Print and shaded views of the part. All mm, measured from the part's lowest x, y and z. A direction names the side the tool comes from. Give positions to 0.01 mm unless a question says otherwise; leave off trailing zeros. Loops run counter-clockwise (first coordinate to the right, second up) from the corner with the lowest first, then second, coordinate; pieces in that order, holes last. Notation, with made-up numbers: (23.25, 59) - (70.25, 59) arc R13 ccw to (70.25, 64) - close; hole circle Ø1 at (-10.75, 44). An arc over 180 degrees is marked (long way). Return JSON: item names as keys, results as strings.
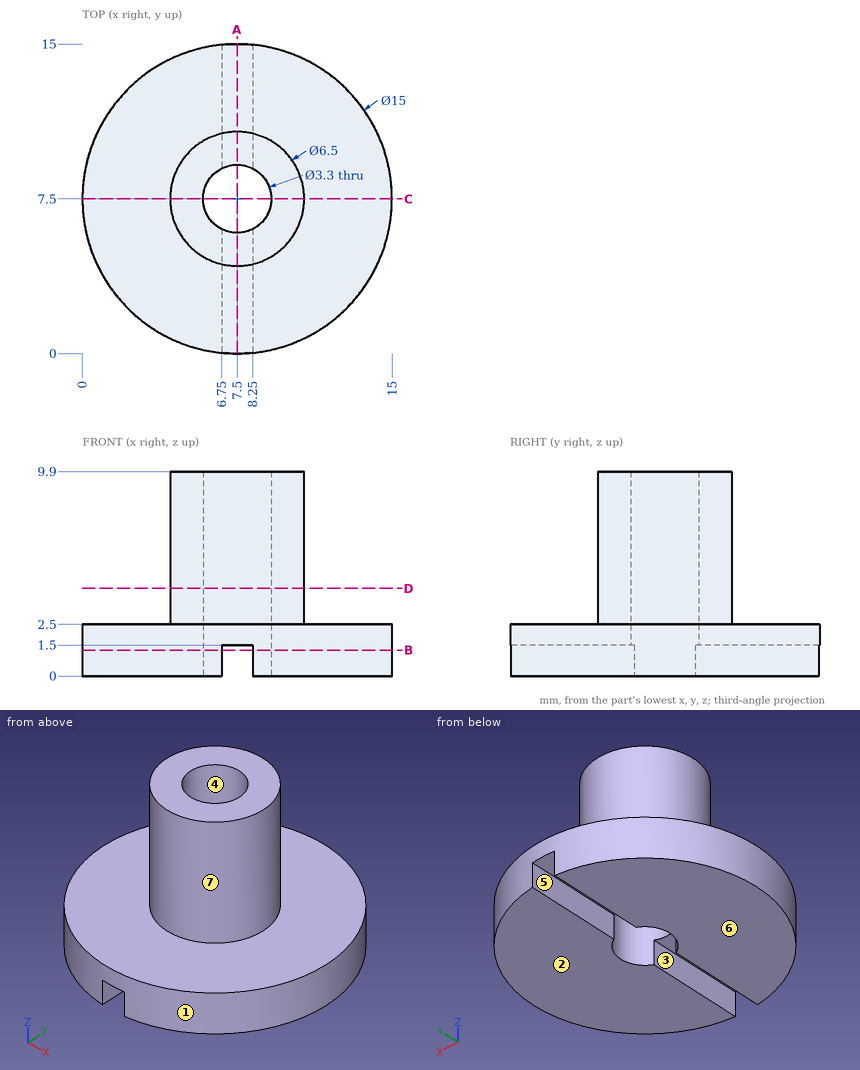
1. Which spindle directions (+Z, -Z, +X, -X, +Y, -Y) get a long thin tool onto all of the face, cutting with end or side? Do the marked faces 5, 6 and 7. Say none if no direction does.
Values follow:
{"face 5": "-Z, +Y, -Y", "face 6": "-Z, +X, -X, +Y, -Y", "face 7": "+Z"}
2. Cut at C-C, the plane y = 7.5. Write the cut outline in (x, z).
Values follow:
{"outline": "(0, 0) - (5.85, 0) - (5.85, 9.9) - (4.25, 9.9) - (4.25, 2.5) - (0, 2.5) - close; (9.15, 0) - (15, 0) - (15, 2.5) - (10.75, 2.5) - (10.75, 9.9) - (9.15, 9.9) - close"}
3. Cut at A-A, the plane x = 7.5. Write the cut outline in (y, z).
Values follow:
{"outline": "(0, 1.5) - (5.85, 1.5) - (5.85, 9.9) - (4.25, 9.9) - (4.25, 2.5) - (0, 2.5) - close; (9.15, 1.5) - (15, 1.5) - (15, 2.5) - (10.75, 2.5) - (10.75, 9.9) - (9.15, 9.9) - close"}
4. Drop flat-ended pins along their axis: P1, Ø0.8, axis at y = 11.5, z = 1, coming from the +X side; P2, Ø0.8, axis at y = 11.5, z = 0.5, coming from the -X side; P3, Ø2, axis at y = 9, z = 6.5, coming from the +X side. Give the stop position or say it passes through.
Values follow:
{"P1": "stops at x = 14.08", "P2": "stops at x = 0.92", "P3": "stops at x = 10.71"}
5. Pull direction X, two halves, no side cores. Call the marked faces 1, 2, 3 and 4: +X half, -X half, draft (parallel to the pull), parting line (faces both ways), or undercut.
Values follow:
{"face 1": "parting line", "face 2": "draft", "face 3": "undercut", "face 4": "undercut"}
6. Cut at D-D, the plane z = 4.25. Write the cut outline in (x, y), plus the area to 3 significant figures.
Values follow:
{"outline": "circle Ø6.5 at (7.5, 7.5); hole circle Ø3.3 at (7.5, 7.5)", "area": "24.6 mm²"}
7. Drill centre lines: probe 1 along Y at (x, z) = (7.5, 5.5); probe 2 along Z at (x, y) = (6.25, 1); probe 3 along Z at (x, y) = (8, 4.5). Where is each one in solid material? Low to high.
Values follow:
{"probe 1": "y = 4.25 to 5.85, 9.15 to 10.75", "probe 2": "z = 0 to 2.5", "probe 3": "z = 1.5 to 9.9"}
8. Cut at B-B, the plane z = 1.25. Write the cut outline in (x, y).
Values follow:
{"outline": "(6.75, 0.04) - (6.75, 6.03) arc R1.65 cw to (6.75, 8.97) - (6.75, 14.96) arc R7.5 ccw to start; (8.25, 0.04) arc R7.5 ccw to (8.25, 14.96) - (8.25, 8.97) arc R1.65 cw to (8.25, 6.03) - close"}
